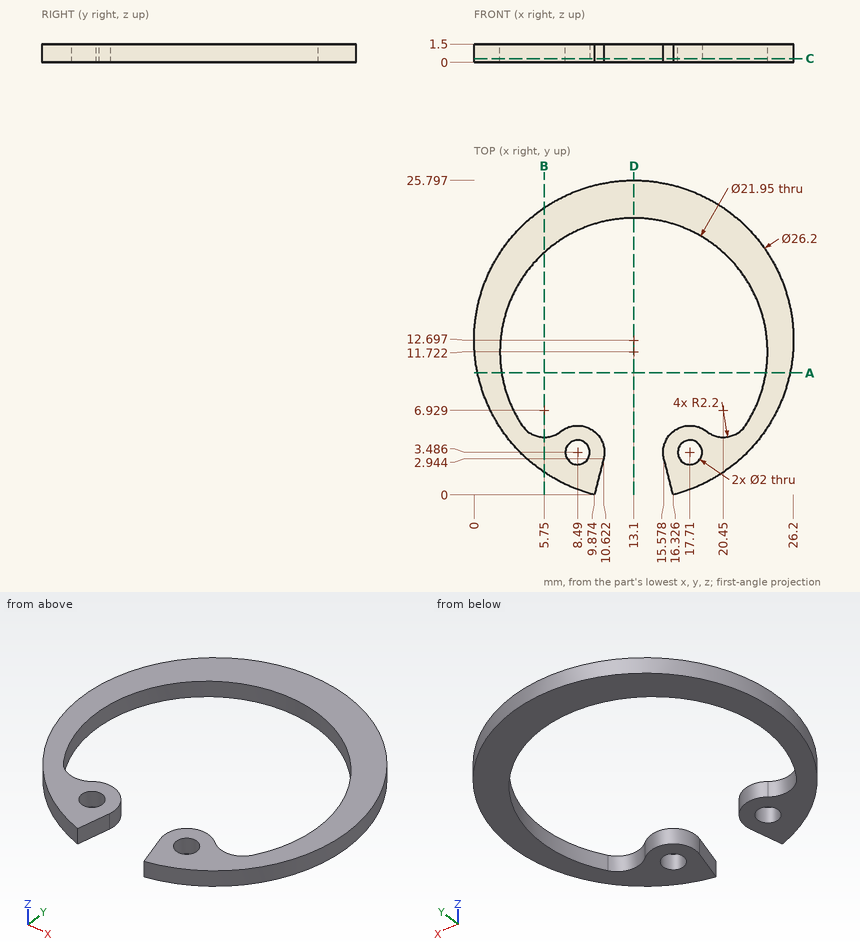
The figure shows three views and two pictorial views of one solid part (mm, origin at its lowest corner). Answer the questions. Round coordinates to 2 decimals unless told otherwise and drop trailing zeros. Write each loop counter-clockwise with the first axis right and the second up, starting at its lowest first coordinate (ties: lowest second). Pieces come first, ordered by that corner, then holes. Notation, with made-up numbers: M 22,78 L 31,78 A24 ccw 31,95 Z; hole C -2.5,64 d8. An arc over 180 degrees is marked long. Use a Markdown table: item, result.
1) The part is cut by section B-B on x = 5.75. Give the vertices of the cut face in (y, z).
Taken from the geometry:
| item | result |
|---|---|
| outline | M 1.85,0 L 4.73,0 L 4.73,1.5 L 1.85,1.5 Z; M 19.87,0 L 23.54,0 L 23.54,1.5 L 19.87,1.5 Z |
2) The part is cut by section A-A on y = 10. Give the vertices of the cut face in (x, z).
Taken from the geometry:
| item | result |
|---|---|
| outline | M 0.28,0 L 2.26,0 L 2.26,1.5 L 0.28,1.5 Z; M 23.94,0 L 25.92,0 L 25.92,1.5 L 23.94,1.5 Z |
3) The part is cut by section C-C on z = 0.3. State how many separate pieces and enclosed holes the cut face has, plus the area to 3 significant figures.
Taken from the geometry:
| item | result |
|---|---|
| separate pieces | 1 |
| enclosed holes | 2 |
| area | 179 mm2 |
4) Consider line 1 (Y direction, x = 18.5, z = 0.6) (1 decimal); line 2 (Y direction, x = 4, z = 0.8) (1 decimal); line 3 (Y direction, x = 22, z = 1) (1 decimal). Determine where each line is inside the solid, lowest interval first. Write a range as [from, to].
Taken from the geometry:
| item | result |
|---|---|
| line 1 | y = [0.8, 2.9], [4.1, 5.5], [21.3, 24.6] |
| line 2 | y = [3.3, 5.6], [17.9, 22.1] |
| line 3 | y = [3.1, 5.4], [18.1, 22.3] |
5) The part is cut by section D-D on x = 13.1. Give the vertices of the cut face in (y, z).
Taken from the geometry:
| item | result |
|---|---|
| outline | M 22.7,0 L 25.8,0 L 25.8,1.5 L 22.7,1.5 Z |
